Study the drawing (mm; zero at the part's minimum x, y, z) and answer. A direction names the side the tool comes from. Round coordinates to 2 decimals unless told otherwise and drop trailing zeros. Write each loop counter-clockwise with the first axis right and the second up, starting at its lowest first coordinate (ties: lowest second). Pieces come first, ordered by that corner, then holes. Notation, with made-up numbers: (86.5, -8.5) -> (100.5, -8.5) arc R29 ccw to (100.5, 19.5) -> close; hole circle Ø2 at (23, 71.5). An arc over 180 degrees is marked (long way). Return JSON: item names as keys, results as strings.
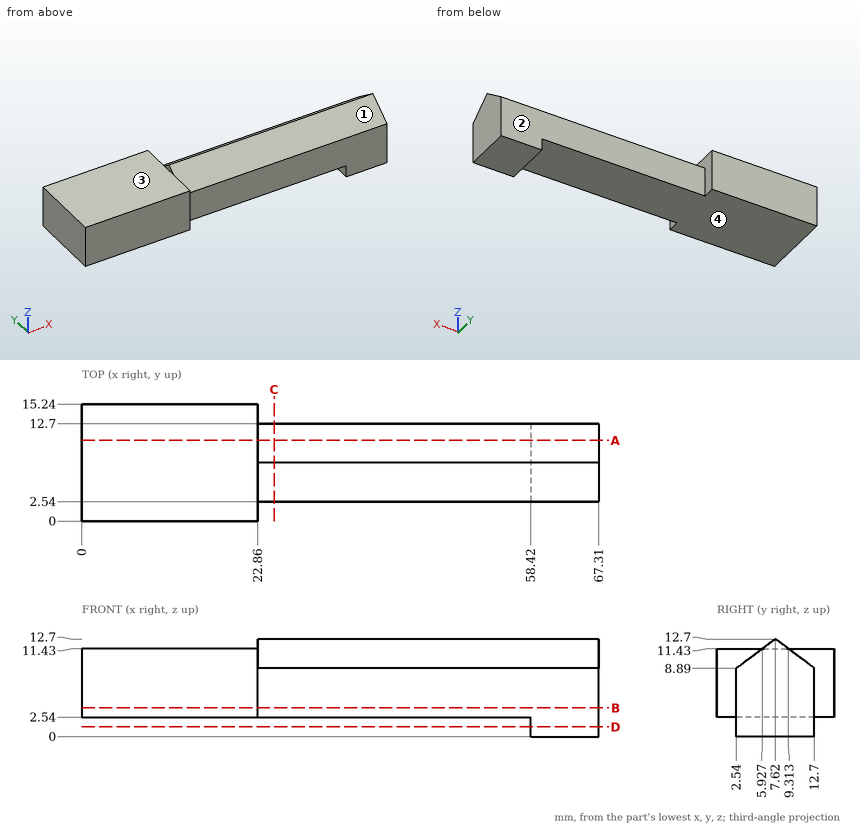
Item 1: A tool of negligible diameter and unlimited length cuts with its end or side. For the marked faces 1, 2, 3 and 4, from which of +Z, -Z, +X, -X, +Y, -Y can it reach the whole face along a straight path? Write none if from no direction.
Worked answers:
{"face 1": "+Z, +X, -Y", "face 2": "+Z, -Z, +X, +Y", "face 3": "+Z, -X, +Y, -Y", "face 4": "-Z, -X, +Y, -Y"}
Item 2: Section C-C (x = 25) is taken. Give the vertices of the cut face in (y, z).
Worked answers:
{"outline": "(2.54, 2.54) -> (12.7, 2.54) -> (12.7, 8.89) -> (7.62, 12.7) -> (2.54, 8.89) -> close"}
Item 3: Straight lines are drawn through the part: L1, parallel to X at y = 8, z = 1.75; L2, parallel to Y at x = 61.5, z = 5.75; L3, parallel to Z at x = 13, y = 4.5. For each, find the intervals that lie inside material, in ascending order. Write a range as [from, to].
Worked answers:
{"L1": "x = [58.42, 67.31]", "L2": "y = [2.54, 12.7]", "L3": "z = [2.54, 11.43]"}
Item 4: Flat-ended cylindrical pins translate along their axes: pin 1 (7.5 mm diameter, centred on x = 24, y = 11, fed in from -Z); pin 2 (4.5 mm diameter, centred on x = 41.5, z = 5.5, fed in from +Y); pin 3 (3 mm diameter, centred on x = 42.5, z = 3.5, fed in from -Y). Find the tip coordinate at first contact, or state that the pin passes through.
Worked answers:
{"pin 1": "stops at z = 2.54", "pin 2": "stops at y = 12.7", "pin 3": "stops at y = 2.54"}
Item 5: Section A-A (y = 10.5) is taken. Give the vertices of the cut face in (x, z).
Worked answers:
{"outline": "(0, 2.54) -> (58.42, 2.54) -> (58.42, 0) -> (67.31, 0) -> (67.31, 10.54) -> (22.86, 10.54) -> (22.86, 11.43) -> (0, 11.43) -> close"}
Item 6: Section B-B (z = 3.75) is taken. Give the vertices of the cut face in (x, y), then the cut area to 3 significant figures.
Worked answers:
{"outline": "(0, 0) -> (22.86, 0) -> (22.86, 2.54) -> (67.31, 2.54) -> (67.31, 12.7) -> (22.86, 12.7) -> (22.86, 15.24) -> (0, 15.24) -> close", "area": "800 mm2"}
Item 7: Section D-D (z = 1.25) is taken. Give the vertices of the cut face in (x, y).
Worked answers:
{"outline": "(58.42, 2.54) -> (67.31, 2.54) -> (67.31, 12.7) -> (58.42, 12.7) -> close"}
